Design review of the part built by this model. Coordinates are the model's own, in mm. Coordinates: 2 decimals unless noted, no trailing zeros. Loops run counter-clockwise (first coordinate to the right, second up) from the corner with the lowest first, then second, coordinate; pieces in that order, holes last. Notation, with made-up numbers: M -1.5,35 L 4.5,35 A16 cw 4.5,43 Z; hole C -16.5,8.5 d1. An arc over 180 degrees is marked long. Put each result on its own line as item: value. Start each with the question number.
(1) Take a section at A-A, the plane y = 0. Give the boundary of the cut face in (x, z) (3 decimals), then the cut area to 3 significant figures.
(2) Take a section at C-C, the plane z = -94. Give the boundary of the cut face in (x, y) (3 decimals), then the cut area to 3 significant figures.
(3) Clearance check with flat-ended pins moving along their axes: pin 1 (4 mm diameter, centred on x = 0, y = 0, fed in from +Z); pin 2 (3 mm diameter, centred on x = 1, y = 0, fed in from -Z); pin 3 (5 mm diameter, centred on x = -4.5, z = -46, fed in from +Y). State where each tip first meets the part, or that it passes through.
(4) Take a section at D-D, the plane z = -22.5. Give the boundary of the cut face in (x, y), then the cut area to 3 significant figures.
(5) For probe 1 along Y at (x, z) = (0, -9.5) (3 decimals); probe 2 along X at (y, z) = (0.25, -41); probe 3 along Z at (x, y) = (2.75, -3), list the stretches that pass through material, from the lowest coordinate up. Write a range as [from, to].
(6) Take a section at B-B, the plane x = 0. Give the boundary of the cut face in (y, z) (3 decimals).
```python
from build123d import *

# Parameters (mm, degrees)
SKETCH1_R               = 6.35
BOSS_EXTRUDE1_DEPTH     = 101.6
SKETCH7_R               = 3.175
CUT_EXTRUDE4_DEPTH      = 12.7
CUT_EXTRUDE5_DEPTH      = 7.62
CUT_EXTRUDE5_DEPTH_BACK = 8.636
SKETCH10_R              = 3.175
CUT_EXTRUDE6_START      = -12.7
SKETCH11_R              = 3.175
CUT_EXTRUDE6_DEPTH      = 12.7


with BuildPart() as part:
    # Sketch1 → Boss-Extrude1 (new body)
    with BuildSketch(Plane.XY):
        Circle(SKETCH1_R)
    extrude(amount=-BOSS_EXTRUDE1_DEPTH)

    # Sketch7 → Cut-Extrude4 (cut)
    with BuildSketch(Plane(origin=(0, 0, -101.6), x_dir=(-1, 0, 0), z_dir=(0, 0, -1))):
        Circle(SKETCH7_R)
    extrude(amount=-CUT_EXTRUDE4_DEPTH, mode=Mode.SUBTRACT)

    # Sketch10 → Cut-Extrude5 (cut, two sides: drawn at the far end of the back side and taken through both)
    with BuildSketch(Plane(origin=(0, 0, 0), x_dir=(1, 0, 0), z_dir=(0, 1, 0)).offset(-CUT_EXTRUDE5_DEPTH_BACK)):
        with Locations(Location((0, 21.844, 0), (0, 0, 90))):
            Circle(SKETCH10_R)
    extrude(amount=CUT_EXTRUDE5_DEPTH + CUT_EXTRUDE5_DEPTH_BACK, mode=Mode.SUBTRACT)

    # Sketch11 → Cut-Extrude6 (cut)
    with BuildSketch(Plane.XY.offset(CUT_EXTRUDE6_START)):
        with Locations(Location((0, 0, 0), (0, 0, 180))):
            Circle(SKETCH11_R)
    extrude(amount=CUT_EXTRUDE6_DEPTH, mode=Mode.SUBTRACT)


solid = part.part
```
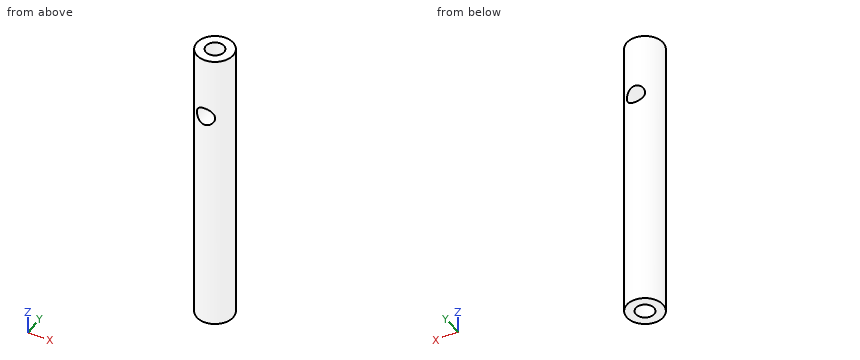
Computed values:
1. outline: M -6.35,-101.6 L -3.175,-101.6 L -3.175,-88.9 L 3.175,-88.9 L 3.175,-101.6 L 6.35,-101.6 L 6.35,0 L 3.175,0 L 3.175,-12.7 L -3.175,-12.7 L -3.175,0 L -6.35,0 Z; hole C 0,-21.844 d6.35
1. area: 1,100 mm^2
2. outline: C 0,0 d12.7; hole C 0,0 d6.35
2. area: 95.0 mm^2
3. pin 1: stops at z = -12.7
3. pin 2: stops at z = -88.9
3. pin 3: stops at y = 6.03
4. outline: M -3.11,-5.54 L -3.11,5.54 A6.35 ccw Z; M 3.11,-5.54 A6.35 ccw 3.11,5.54 Z
4. area: 51.0 mm^2
5. probe 1: y = [-6.35, -3.175], [3.175, 6.35]
5. probe 2: x = [-6.35, 6.35]
5. probe 3: z = [-101.6, -23.43], [-20.26, 0]
6. outline: M -6.35,-101.6 L -3.175,-101.6 L -3.175,-88.9 L 3.175,-88.9 L 3.175,-101.6 L 6.35,-101.6 L 6.35,-25.019 L -6.35,-25.019 Z; M -6.35,-18.669 L 6.35,-18.669 L 6.35,0 L 3.175,0 L 3.175,-12.7 L -3.175,-12.7 L -3.175,0 L -6.35,0 Z
